Can you work these out from the model? Positions are in its coordinate system, mm. Give positions to 0.01 mm unless a question says otherwise; leave off trailing zeros. Order: outer loops, then holes, each group sorted by start corner. A loop starts at its lowest first (then second) coordinate and runs counter-clockwise, first axis right, second up. Notation, with made-up numbers: (82.25, 63) - (126.25, 63) arc R24 cw to (126.25, 73) - close; hole circle Ø2 at (11, -3). An arc over 180 degrees is marked (long way). One line per question, with ' | ' between items.
```python
from build123d import *

# Parameters (mm, degrees)
F1_DEPTH = 79
F2_R     = 1.5


with BuildPart() as f1:
    # F0 (on Front) → F1 (new body)
    with BuildSketch(Plane.XZ):
        with BuildLine():
            Line((33.5, 3), (-33.5, 3))
            ThreePointArc((-33.5, 3), (-34.56066, 2.56066), (-35, 1.5))
            Line((-35, 1.5), (-35, -1))
            ThreePointArc((-35, -1), (0, 0), (35, -1))
            Line((35, -1), (35, 1.5))
            ThreePointArc((35, 1.5), (34.56066, 2.56066), (33.5, 3))
        make_face()
    extrude(amount=F1_DEPTH)

    # F2
    f2_edges = [f1.edges().sort_by_distance(p)[0] for p in [
        (33.5, -39.5, 3),
        (35, -39.5, 1.5),
        (34.56066, 0, 2.56066),
        (34.56066, -79, 2.56066),
    ]]
    fillet(f2_edges, radius=F2_R)


solid = f1.part
```
(1) Imagine slicing it at B-B (y = -52). List the corners of the cut face in (x, z) for me.
Answer below:
outline: (-35, -1) arc R613 cw to (35, -1) - (35, 1.5) arc R1.5 ccw to (33.5, 3) - (-33.5, 3) arc R1.5 ccw to (-35, 1.5) - close
(2) Imagine slicing it at A-A (x = 24). List the corners of the cut face in (y, z) for me, and give its area (3 significant figures).
Answer below:
outline: (-79, -0.47) - (0, -0.47) - (0, 1.5) arc R1.5 ccw to (-1.5, 3) - (-77.5, 3) arc R1.5 ccw to (-79, 1.5) - close | area: 273 mm^2
(3) Will these pins go through, and if not, where does the flat tip stop? pin 1 (5 mm diameter, centred on x = 19, y = -46.5, fed in from -Z); pin 2 (12 mm diameter, centred on x = 10.5, y = -52, fed in from -Z); pin 3 (2 mm diameter, centred on x = -18.5, y = -47, fed in from -Z).
Answer below:
pin 1: z = -0.38 | pin 2: z = -0.22 | pin 3: z = -0.31
(4) If I drill on line 1 (Y direction, x = 6, z = 1.7); line 2 (Z direction, x = 3, y = -11); line 3 (Z direction, x = 18, y = -37.5), over which ranges is the centre line in solid material (lowest first)?
Answer below:
line 1: -78.99 to -0.01 | line 2: -0.01 to 3 | line 3: -0.26 to 3
